from build123d import *

# Parameters (mm, degrees)
BOSS_EXTRUDE1_DEPTH = 1.524


with BuildPart() as part:
    # Sketch1 → Boss-Extrude1 (new body)
    with BuildSketch(Plane.XY):
        with BuildLine():
            Line((-229.733299104, 584.719331839), (-222.502527935, 583.634973996))
            ThreePointArc((-222.502527935, 583.634973996), (-221.147267888, 584.004051618), (-220.092288362, 584.931395291))
            ThreePointArc((-220.092288362, 584.931395291), (-219.107825608, 581.890435474), (-219.721109978, 578.753480613))
            Line((-219.721109978, 578.753480613), (-228.459709631, 579.934984791))
            Line((-228.459709631, 579.934984791), (-228.661688518, 578.44207641))
            Line((-228.661688518, 578.44207641), (-220.092288362, 577.283710625))
            ThreePointArc((-220.092288362, 577.283710625), (-221.51932816, 574.510272261), (-222.100657588, 571.445886672))
            ThreePointArc((-222.100657588, 571.445886672), (-226.629664964, 572.833617667), (-231.313271906, 573.541806308))
            ThreePointArc((-231.313271906, 573.541806308), (-233.223508643, 573.597615767), (-235.134519327, 573.610155801))
            ThreePointArc((-235.134519327, 573.610155801), (-234.714498742, 572.38977797), (-233.834266637, 571.445886672))
            ThreePointArc((-233.834266637, 571.445886672), (-238.740309086, 572.778591559), (-243.812582366, 573.121226369))
            ThreePointArc((-243.812582366, 573.121226369), (-249.654593018, 572.281403909), (-255.423617198, 571.035309918))
            ThreePointArc((-255.423617198, 571.035309918), (-254.208732466, 570.049679285), (-252.813402451, 569.342242498))
            ThreePointArc((-252.813402451, 569.342242498), (-257.023373112, 569.616476447), (-261.233343772, 569.342242498))
            ThreePointArc((-261.233343772, 569.342242498), (-262.139462052, 569.036834334), (-263.042061741, 568.721179006))
            ThreePointArc((-263.042061741, 568.721179006), (-265.382908747, 568.898961953), (-266.820790496, 570.754674096))
            ThreePointArc((-266.820790496, 570.754674096), (-267.633321548, 574.021224174), (-268.462018281, 577.283710625))
            ThreePointArc((-268.462018281, 577.283710625), (-269.684214588, 576.035290864), (-271.430597221, 575.985658132))
            ThreePointArc((-271.430597221, 575.985658132), (-270.077505732, 579.055656064), (-269.795996664, 582.398782822))
            ThreePointArc((-269.795996664, 582.398782822), (-270.6063104, 585.428884975), (-271.430597221, 588.455215862))
            ThreePointArc((-271.430597221, 588.455215862), (-272.402462147, 590.846491133), (-273.540779849, 593.163159358))
            ThreePointArc((-273.540779849, 593.163159358), (-274.047233126, 591.694203826), (-275.473581255, 591.077878999))
            ThreePointArc((-275.473581255, 591.077878999), (-275.34428452, 594.597865441), (-276.57079113, 597.899789688))
            ThreePointArc((-276.57079113, 597.899789688), (-280.26245264, 602.086630283), (-284.548965797, 605.662074848))
            ThreePointArc((-284.548965797, 605.662074848), (-285.652879269, 603.854761803), (-285.375456051, 601.755228103))
            ThreePointArc((-285.375456051, 601.755228103), (-289.30709222, 606.735438718), (-294.333091655, 610.608369187))
            ThreePointArc((-294.333091655, 610.608369187), (-296.477583287, 611.240889296), (-298.65675661, 611.741018952))
            ThreePointArc((-298.65675661, 611.741018952), (-302.990086346, 612.65022374), (-306.51096198, 615.334964829))
            ThreePointArc((-306.51096198, 615.334964829), (-302.406354647, 614.521452362), (-298.222601436, 614.597695151))
            ThreePointArc((-298.222601436, 614.597695151), (-285.35767493, 610.750777653), (-274.736325292, 602.53542373))
            ThreePointArc((-274.736325292, 602.53542373), (-269.209056442, 598.616541826), (-265.187992407, 593.163159358))
            ThreePointArc((-265.187992407, 593.163159358), (-267.353928299, 594.342358031), (-269.657730455, 595.222291793))
            ThreePointArc((-269.657730455, 595.222291793), (-268.234509905, 592.198490903), (-267.092140084, 589.057803121))
            ThreePointArc((-267.092140084, 589.057803121), (-266.592090958, 587.698505955), (-266.111218097, 586.33230714))
            ThreePointArc((-266.111218097, 586.33230714), (-263.083103018, 583.668794976), (-259.392672976, 582.04260185))
            ThreePointArc((-259.392672976, 582.04260185), (-261.970528382, 581.721095666), (-264.339245348, 580.654378901))
            ThreePointArc((-264.339245348, 580.654378901), (-263.715375229, 578.327001479), (-263.146155659, 575.985658132))
            ThreePointArc((-263.146155659, 575.985658132), (-262.422892661, 575.037653784), (-261.233343772, 574.955221701))
            ThreePointArc((-261.233343772, 574.955221701), (-251.134066148, 577.939069272), (-240.721980879, 579.516166347))
            ThreePointArc((-240.721980879, 579.516166347), (-237.604479811, 584.0033655), (-232.878306602, 586.745090494))
            ThreePointArc((-232.878306602, 586.745090494), (-234.104874481, 585.261460478), (-235.134519327, 583.634973996))
            ThreePointArc((-235.134519327, 583.634973996), (-232.495519695, 584.484036639), (-229.733299104, 584.719331839))
        make_face()
    extrude(amount=BOSS_EXTRUDE1_DEPTH)


solid = part.part
CAD build for the part. Positions are in the model's coordinates, mm. A direction names the side the tool comes from. Round coordinates to 2 decimals unless told otherwise and drop trailing zeros. Order: outer loops, then holes, each group sorted by start corner. A loop starts at its lowest first (then second) coordinate and runs counter-clockwise, first axis right, second up. Notation, with made-up numbers: (41.5, 1.25) -> (59.5, 1.25) arc R27 cw to (59.5, 39.25) -> close; hole circle Ø5 at (40, 41). An arc over 180 degrees is marked (long way). Write each question's results on one line, items separated by ' | '.
1. Pull direction X, two halves, no side cores. Call faces 4 (the face through (-289.24, 606.67, 0.75)), 5 (the face through (-285.53, 610.84, 0.75)), 6 (the face through (-280.206, 602.032, 0.751)): pulls with the +X half, pulls with the -X half, needs draft (parallel to the pull), parting line crosses it, or undercut.
Findings below:
face 4: pulls with the -X half | face 5: pulls with the +X half | face 6: undercut
2. Cut at B-B (y = 600). Give the cut face in (x, z), plus the area to 3 significant figures.
Findings below:
outline: (-278.28, 0) -> (-270.76, 0) -> (-270.76, 1.52) -> (-278.28, 1.52) -> close | area: 11.5 mm²
3. Wall check: line 1 along X through (y, z) = (585.5, 0.2); line 2 along X through (y, z) = (581, 0.6); line 3 along Y through (x, z) = (-249, 0.1). Give the ranges that are in metal, low to high. Write a range as [from, to].
Findings below:
line 1: x = [-270.63, -265.35], [-235.62, -233.93] | line 2: x = [-269.78, -263.75], [-240, -219.12] | line 3: y = [572.4, 578.38]
4. Cut at A-A (x = -249.5). Give the cut face in (y, z).
Findings below:
outline: (572.31, 0) -> (578.28, 0) -> (578.28, 1.52) -> (572.31, 1.52) -> close
5. 3-axis set-ups, long thin cutter, end or side, ignore diameter. For faces 1 (the face through (-228.56, 579.2, 0.75)), 2 (the face through (-237.66, 583.95, 0.75)), 3 (the face through (-270.09, 579.01, 0.75)): which of +Z, -Z, +X, -X, +Y, -Y reach the whole face in a straight line?
Findings below:
face 1: +Z, -Z | face 2: +Z, -Z, +Y | face 3: +Z, -Z, -X
